Design review of the part built by this model. Coordinates are the model's own, in mm. A direction names the side the tool comes from. Give positions to 0.01 mm unless a question says otherwise; leave off trailing zeros. Order: outer loops, then holes, each group sorted by start corner. A loop starts at its lowest first (then second) coordinate and runs counter-clockwise, first axis right, second up. Notation, with made-up numbers: (40, 54.5) -> (67, 54.5) arc R8 ccw to (67, 68.5) -> close; hole circle Ø7 at (88.5, -18). An arc over 180 degrees is marked (long way). Use a Markdown table: item, result. Add a question column.
```python
from build123d import *

# Parameters (mm, degrees)
CHANFREIN1_SIZE                                    = 0.5
CHAMBRAGE_POUR_VIS_T_TE_HEXAGONALE_M41_D           = 4.5
CHAMBRAGE_POUR_VIS_T_TE_HEXAGONALE_M41_CBORE_D     = 8
CHAMBRAGE_POUR_VIS_T_TE_HEXAGONALE_M41_CBORE_DEPTH = 4.4
ENL_V_MAT_EXTRU_2_DEPTH                            = 130.336769714
CHANFREIN3_SIZE                                    = 0.5
ESQUISSE12_W                                       = 3
ESQUISSE12_H                                       = 11.621091342
ENL_V_MAT_EXTRU_3_DEPTH                            = 3
D_GAGEMENT_M21_D                                   = 2.4
D_GAGEMENT_M21_DEPTH                               = 5
D_GAGEMENT_M21_TIP                                 = 0.692820323


with BuildPart() as part:
    # Esquisse1 → Révolution1 (revolve)
    with BuildSketch(Plane.XY):
        Polygon((15, 6), (124, 6), (124, 0), (0, 0), (0, 26), (6, 26), (6, 10), (15, 10), align=None)
    revolve(axis=Axis((124, 0, 0), (-1, 0, 0)))

    # Chanfrein1
    chanfrein1_edges = [part.edges().sort_by_distance(p)[0] for p in [
        (6, -26, 0),
        (15, -10, 0),
    ]]
    chamfer(chanfrein1_edges, length=CHANFREIN1_SIZE)

    # Chambrage pour vis à tête hexagonale M41 (through all)
    with Locations(Plane(origin=(6, 0, 0), x_dir=(0, 0, -1), z_dir=(1, 0, 0))):
        with Locations((-21, 0), (21, 0)):
            CounterBoreHole(CHAMBRAGE_POUR_VIS_T_TE_HEXAGONALE_M41_D / 2, CHAMBRAGE_POUR_VIS_T_TE_HEXAGONALE_M41_CBORE_D / 2, CHAMBRAGE_POUR_VIS_T_TE_HEXAGONALE_M41_CBORE_DEPTH)

    # Esquisse11 → Enlèv. mat.-Extru.2 (cut, through all)
    with BuildSketch(Plane.ZY):
        with BuildLine():
            Line((24, -10), (-24, -10))
            ThreePointArc((-24, -10), (0, -26), (24, -10))
        make_face()
        with BuildLine():
            Line((24, 10), (-24, 10))
            ThreePointArc((-24, 10), (0, 26), (24, 10))
        make_face()
    extrude(amount=-ENL_V_MAT_EXTRU_2_DEPTH, mode=Mode.SUBTRACT)

    # Chanfrein3
    chanfrein3_edges = [part.edges().sort_by_distance(p)[0] for p in [
        (124, -6, 0),
    ]]
    chamfer(chanfrein3_edges, length=CHANFREIN3_SIZE)

    # Esquisse12 → Enlèv. mat.-Extru.3 (cut)
    with BuildSketch(Plane(origin=(124, 0, 0), x_dir=(0, 0, -1), z_dir=(1, 0, 0))):
        with Locations((0, -3.191920072)):
            Rectangle(ESQUISSE12_W, ESQUISSE12_H)
    extrude(amount=-ENL_V_MAT_EXTRU_3_DEPTH, mode=Mode.SUBTRACT)

    # Dégagement M21
    with Locations(Plane(origin=(121, 0, 0), x_dir=(0, 0, -1), z_dir=(1, 0, 0))):
        with Locations((0, 0), (0, -3.724850959)):
            Hole(D_GAGEMENT_M21_D / 2, depth=D_GAGEMENT_M21_DEPTH)
            with Locations((0, 0, -(D_GAGEMENT_M21_DEPTH + D_GAGEMENT_M21_TIP / 2))):  # 120° drill point
                Cone(0, D_GAGEMENT_M21_D / 2, D_GAGEMENT_M21_TIP, mode=Mode.SUBTRACT)


solid = part.part
```
1) Machinability: for faces 5 (the flat face through (123, -2, -1.5)), 6 (the cylindrical face through (3.8, -2.4, -17.8)), 7 (the flat face through (124, 0, 2)), which of the approach directions +Z, -Z, +X, -X, +Y, -Y give a long, thin tool a straight path to every point of the face, cutting with its end or side? Answer none if there is none.
2) Add section B-B (x = 60). Give the boundary of the cut face in (y, z), then the cut area to 3 significant figures.
3) The part is to be moulded in two halves that separate along Z. For faces 1 (the cylindrical face through (118.465, -4.896, -0.26)), 2 (the conical face through (5.865, -0.145, 25.635)), 3 (the cylindrical face through (3, 0, -26)), 4 (the conical face through (115.43, -3.93, 0.05)), say which applies: +Z half, -Z half, draft (parallel to the pull), parting line (faces both ways), or undercut.
4) Add section A-A (z = -21). Give the boundary of the cut face in (x, y).
5) For L1, parallel to Y at x = 119.25, z = 0; L2, parallel to Z at x = 117.65, y = 0; L3, parallel to Y at x = 3.9, z = -21, list the stretches that pass through material, from the lowest coordinate up. Write a range as [from, to].
6) Add section C-C (z = -14). Give the boundary of the cut face in (x, y).
7) Insertion check: pin 1 (6 mm diameter, centred on y = 1.5, z = 12.5, fed in from +X); pin 2 (1.5 mm diameter, centred on x = 122, y = -1.5, fed in from +Z); pin 3 (1.5 mm diameter, centred on x = 21.5, y = -2, fed in from +Z). Each pin has a flat end and moves straight along its axis. Give the tip position at first contact, or say it passes through.
Worked answers:
| question | item | result |
|---|---|---|
| 1 | face 5 | +X, -Y |
| 1 | face 6 | +X |
| 1 | face 7 | +Z, -Z, +X, +Y, -Y |
| 2 | outline | circle Ø12 at (0, 0) |
| 2 | area | 113 mm^2 |
| 3 | face 1 | undercut |
| 3 | face 2 | +Z half |
| 3 | face 3 | -Z half |
| 3 | face 4 | undercut |
| 4 | outline | (0, -10) -> (6, -10) -> (6, -4) -> (1.6, -4) -> (1.6, -2.25) -> (0, -2.25) -> close; (0, 2.25) -> (1.6, 2.25) -> (1.6, 4) -> (6, 4) -> (6, 10) -> (0, 10) -> close |
| 5 | L1 | [-6, -4.92], [-2.52, -1.2], [1.2, 6] |
| 5 | L2 | [-6, -1.2], [1.2, 6] |
| 5 | L3 | [-10, -4], [4, 10] |
| 6 | outline | (0, -10) -> (6, -10) -> (6, 10) -> (0, 10) -> close |
| 7 | pin 1 | x = 14.91 |
| 7 | pin 2 | z = 5.95 |
| 7 | pin 3 | z = 5.87 |
